```python
from build123d import *

# Parameters (mm, degrees)
SKIZZE1_R                       = 12
SKIZZE1_R_2                     = 1.5
AUFSATZ_LINEAR_AUSTRAGEN1_DEPTH = 17
SKIZZE2_R                       = 3.1
SCHNITT_LINEAR_AUSTRAGEN2_DEPTH = 12


with BuildPart() as part:
    # Skizze1 → Aufsatz-Linear austragen1 (new body)
    with BuildSketch(Plane.XY):
        Circle(SKIZZE1_R)
        with Locations((6.363961031, 6.363961031)):
            Circle(SKIZZE1_R_2, mode=Mode.SUBTRACT)
        with Locations((-6.363961031, 6.363961031)):
            Circle(SKIZZE1_R_2, mode=Mode.SUBTRACT)
        with Locations((-6.363961031, -6.363961031)):
            Circle(SKIZZE1_R_2, mode=Mode.SUBTRACT)
        with Locations((6.363961031, -6.363961031)):
            Circle(SKIZZE1_R_2, mode=Mode.SUBTRACT)
        with BuildLine():
            ThreePointArc((3.795721275, -1.55), (-4.1, 0), (3.795721275, 1.55))
            Line((3.795721275, 1.55), (5.2, 1.55))
            Line((5.2, 1.55), (5.2, -1.55))
            Line((5.2, -1.55), (3.795721275, -1.55))
        make_face(mode=Mode.SUBTRACT)
    extrude(amount=AUFSATZ_LINEAR_AUSTRAGEN1_DEPTH)

    # Skizze2 → Schnitt-Linear austragen2 (cut)
    with BuildSketch(Plane.XY.offset(17)):
        with Locations((-6.363961031, 6.363961031)):
            Circle(SKIZZE2_R)
        with Locations((6.363961031, 6.363961031)):
            Circle(SKIZZE2_R)
        with Locations((6.363961031, -6.363961031)):
            Circle(SKIZZE2_R)
        with Locations((-6.363961031, -6.363961031)):
            Circle(SKIZZE2_R)
    extrude(amount=-SCHNITT_LINEAR_AUSTRAGEN2_DEPTH, mode=Mode.SUBTRACT)


solid = part.part
```
CAD build for the part. Positions are in the model's coordinates, mm. A direction names the side the tool comes from. Round coordinates to 2 decimals unless told otherwise and drop trailing zeros. Order: outer loops, then holes, each group sorted by start corner. A loop starts at its lowest first (then second) coordinate and runs counter-clockwise, first axis right, second up.
Q1. Two-plate mould, pull along X, no slides. Class faces 4 (the flat face through (0, -5, 17)), 5 (the cylindrical face through (5.537, -10.646, 8.381)), 6 (the cylindrical face through (4.261, -4.086, 11.084)): pulls with the +X half, pulls with the -X half, needs draft (parallel to the pull), parting line crosses it, or undercut.
Q2. Slice it at D-D (x = 1). Write the cut outline in (y, z), and give its area (3 significant figures).
Q3. Slice it at C-C (z = 10.5). Write the cut outline in (x, y).
Q4. Which spindle directions (+Z, -Z, +X, -X, +Y, -Y) get a long thin tool onto all of the face, cutting with end or side? Do faces 1 (the flat face through (6, -8, 5)), 2 (the flat face through (4, 1.55, 8)), 3 (the flat face through (0, -5, 0)). Say none if no direction does.
Q5. Wall check: L1, parallel to X at y = -5.5, z = 2; L2, parallel to X at y = -5, z = 14; L3, parallel to Y at x = 5.75, z = 4.75. Give the ranges that are in metal, low to high.
Q6. Slice it at A-A (y = 0). Write the cut outline in (x, z), and give its area (3 significant figures).
Q7. Drop flat-ended pins along their axis: pin 1 (3 mm diameter, centred on x = 5, y = 6, fed in from +Z); pin 2 (1.5 mm diameter, centred on x = 5.5, z = 15.5, fed in from -Y); pin 3 (1.1 mm diameter, centred on x = 4.5, z = 6.5, fed in from +Y). Give the stop position or say it passes through.
Q8. Slice it at B-B (x = 6.75). Write the cut outline in (y, z).
Results below:
1. face 4: needs draft
1. face 5: parting line crosses it
1. face 6: undercut
2. outline: (-11.96, 0) - (-3.98, 0) - (-3.98, 17) - (-11.96, 17) - close; (3.98, 0) - (11.96, 0) - (11.96, 17) - (3.98, 17) - close
2. area: 271 mm2
3. outline: (-9.1, -7.82) arc R3.1 cw (long way) to (-7.82, -9.1) arc R12 ccw to (7.82, -9.1) arc R3.1 cw (long way) to (9.1, -7.82) arc R12 ccw to (9.1, 7.82) arc R3.1 cw (long way) to (7.82, 9.1) arc R12 ccw to (-7.82, 9.1) arc R3.1 cw (long way) to (-9.1, 7.82) arc R12 ccw to start; hole (3.8, -1.55) - (5.2, -1.55) - (5.2, 1.55) - (3.8, 1.55) arc R4.1 ccw (long way) to start
4. face 1: +Z
4. face 2: +Z, -Z
4. face 3: -Z, +X, -X, +Y, -Y
5. L1: x = -10.67 to -7.59, -5.14 to 5.14, 7.59 to 10.67
5. L2: x = -10.91 to -9.15, -3.58 to 3.58, 9.15 to 10.91
5. L3: y = -10.53 to -7.73, -5 to 5, 7.73 to 10.53
6. outline: (-12, 0) - (-4.1, 0) - (-4.1, 17) - (-12, 17) - close; (5.2, 0) - (12, 0) - (12, 17) - (5.2, 17) - close
6. area: 250 mm2
7. pin 1: stops at z = 5
7. pin 2: stops at y = -11.02
7. pin 3: stops at y = 11.33
8. outline: (-9.92, 0) - (-7.81, 0) - (-7.81, 5) - (-9.44, 5) - (-9.44, 17) - (-9.92, 17) - close; (-4.91, 0) - (4.91, 0) - (4.91, 5) - (3.29, 5) - (3.29, 17) - (-3.29, 17) - (-3.29, 5) - (-4.91, 5) - close; (7.81, 0) - (9.92, 0) - (9.92, 17) - (9.44, 17) - (9.44, 5) - (7.81, 5) - close
